Source: CAD feature listing. Evaluate the final solid. Frame: model axes, mm. Face numbers are marked on the shaded views. A direction names the side the tool comes from. Round coordinates to 2 decimals unless told otherwise and drop trailing zeros. Write each loop counter-clockwise with the first axis right and the second up, starting at its lowest first coordinate (ties: lowest second). Pieces come first, ordered by that corner, then holes.
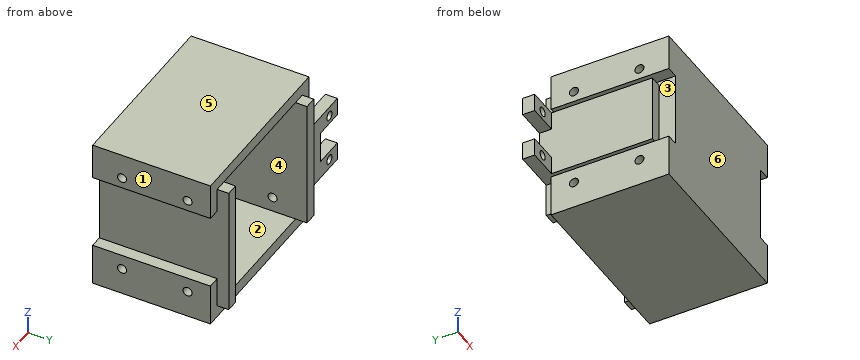
```python
from build123d import *

# Parameters (mm, degrees)
BOSS_EXTRUDE1_DEPTH      = 43
SKETCH4_W                = 50.5
SKETCH4_H                = 39.147537046
BOSS_EXTRUDE2_DEPTH      = 4
SKETCH5_W                = 50.5
SKETCH5_H                = 39.147537046
BOSS_EXTRUDE3_DEPTH      = 4
BOSS_EXTRUDE4_DEPTH      = 17.5
BOSS_EXTRUDE4_DEPTH_BACK = 16
BOSS_EXTRUDE5_START      = 17.5
SKETCH3_3_W              = 10
SKETCH3_3_H              = 6
SKETCH3_3_R              = 1.5
BOSS_EXTRUDE5_DEPTH      = 4
BOSS_EXTRUDE5_2_DEPTH    = 4
BOSS_EXTRUDE6_START      = 17.5
BOSS_EXTRUDE6_DEPTH      = 4
BOSS_EXTRUDE7_DEPTH      = 4
BOSS_EXTRUDE7_DEPTH_BACK = 10
SKETCH5_3_W              = 4
SKETCH5_3_H              = 39.147537046
BOSS_EXTRUDE8_DEPTH      = 4
BOSS_EXTRUDE8_DEPTH_BACK = 8
SKETCH8_R                = 1.5
CUT_EXTRUDE1_DEPTH       = 79.060873682
SKETCH11_R               = 1.5
CUT_EXTRUDE2_DEPTH       = 79.060873682


with BuildPart() as part:
    # Sketch1 → Boss-Extrude1 (new body)
    with BuildSketch(Plane.XY):
        Polygon((-21.25, -17.493697991), (-21.25, 21.493697991), (-25.25, 21.493697991), (-25.25, -21.493697991), (25.25, -21.493697991), (25.25, 21.493697991), (21.25, 21.493697991), (21.25, -17.493697991), align=None)
    extrude(amount=BOSS_EXTRUDE1_DEPTH)

    # Sketch4 → Boss-Extrude2 (add)
    with BuildSketch(Plane.XY.offset(43)):
        with Locations((0, -1.919929468)):
            Rectangle(SKETCH4_W, SKETCH4_H)
    extrude(amount=BOSS_EXTRUDE2_DEPTH)

    # Sketch5 → Boss-Extrude3 (add)
    with BuildSketch(Plane(origin=(0, 0, 0), x_dir=(-1, 0, 0), z_dir=(0, 0, -1))):
        with Locations((0, -1.919929468)):
            Rectangle(SKETCH5_W, SKETCH5_H)
    extrude(amount=BOSS_EXTRUDE3_DEPTH)


with BuildPart() as boss_extrude4_tool:
    # Sketch3 → Boss-Extrude4 (new, two sides: drawn at the far end of the back side and taken through both)
    with BuildSketch(Plane(origin=(0, 0, 0), x_dir=(1, 0, 0), z_dir=(0, 1, 0)).offset(-BOSS_EXTRUDE4_DEPTH_BACK)):
        Polygon((-29.250003781, -33.625807881), (-25.250003781, -33.625807881), (-25.250003781, -11.171909281), (-29.250003781, -11.171909281), (-29.250003781, -17.171909281), (-29.250003781, -27.625807881), align=None)
    extrude(amount=BOSS_EXTRUDE4_DEPTH + BOSS_EXTRUDE4_DEPTH_BACK)


with BuildPart() as part_1:
    add(part.part)


with BuildPart() as part_2:
    # Boss-Extrude4: joined with boss_extrude4_tool
    add(part_1.part.fuse(boss_extrude4_tool.part, tol=0.00001))


with BuildPart() as body_2:
    # Sketch3<3> → Boss-Extrude5 (new body)
    with BuildSketch(Plane(origin=(0, 0, 0), x_dir=(1, 0, 0), z_dir=(0, 1, 0)).offset(BOSS_EXTRUDE5_START)):
        with Locations((-34.250003781, -30.625807881)):
            Rectangle(SKETCH3_3_W, SKETCH3_3_H)
        with Locations(Location((-34.536906803, -30.406566851, 0), (0, 0, 270))):
            Circle(SKETCH3_3_R, mode=Mode.SUBTRACT)
    extrude(amount=BOSS_EXTRUDE5_DEPTH)


with BuildPart() as body_3:
    # Sketch3<3> → Boss-Extrude5 2 (new body)
    with BuildSketch(Plane(origin=(0, 0, 0), x_dir=(1, 0, 0), z_dir=(0, 1, 0)).offset(BOSS_EXTRUDE5_START)):
        with Locations((-34.250003781, -14.171909281)):
            Rectangle(SKETCH3_3_W, SKETCH3_3_H)
        with Locations(Location((-34.536906803, -14.310361699, 0), (0, 0, 270))):
            Circle(SKETCH3_3_R, mode=Mode.SUBTRACT)
    extrude(amount=BOSS_EXTRUDE5_2_DEPTH)


with BuildPart() as boss_extrude6_tool:
    # Sketch3<4> → Boss-Extrude6 (new body)
    with BuildSketch(Plane(origin=(0, 0, 0), x_dir=(1, 0, 0), z_dir=(0, 1, 0)).offset(BOSS_EXTRUDE6_START)):
        Polygon((-29.250003781, -33.625807881), (-25.250003781, -33.625807881), (-25.250003781, -11.171909281), (-29.250003781, -11.171909281), (-29.250003781, -17.171909281), (-29.250003781, -27.625807881), align=None)
    extrude(amount=BOSS_EXTRUDE6_DEPTH)


with BuildPart() as part_3:
    add(part_2.part)


with BuildPart() as part_4:
    # Boss-Extrude6: joined with boss_extrude6_tool
    add(part_3.part.fuse(boss_extrude6_tool.part, body_2.part, body_3.part, tol=0.00001))

    # Sketch5<3> → Boss-Extrude7 (add, two sides: drawn at the far end of the back side and taken through both)
    with BuildSketch(Plane(origin=(0, 0, 0), x_dir=(-1, 0, 0), z_dir=(0, 0, -1)).offset(-BOSS_EXTRUDE7_DEPTH_BACK)):
        with Locations((-27.25, -1.919929468)):
            Rectangle(SKETCH5_3_W, SKETCH5_3_H)
        with Locations((27.25, -1.919929468)):
            Rectangle(SKETCH5_3_W, SKETCH5_3_H)
    extrude(amount=BOSS_EXTRUDE7_DEPTH + BOSS_EXTRUDE7_DEPTH_BACK)

    # Sketch4<3> → Boss-Extrude8 (add, two sides: drawn at the far end of the back side and taken through both)
    with BuildSketch(Plane.XY.offset(43).offset(-BOSS_EXTRUDE8_DEPTH_BACK)):
        Polygon((29.25, 17.653839055), (25.25, 17.653839055), (25.25, -21.493697991), (29.25, -21.493697991), (29.25, -17.493697991), (29.25, 13.653839055), align=None)
        Polygon((-25.25, -21.493697991), (-25.25, 17.653839055), (-29.25, 17.653839055), (-29.25, 13.653839055), (-29.25, -17.493697991), (-29.25, -21.493697991), align=None)
    extrude(amount=BOSS_EXTRUDE8_DEPTH + BOSS_EXTRUDE8_DEPTH_BACK)

    # Sketch8 → Cut-Extrude1 (cut, through all)
    with BuildSketch(Plane.ZY.offset(29.25)):
        with Locations((5.005736184, 10.04444872)):
            Circle(SKETCH8_R)
        with Locations((5.005736184, -11.726773354)):
            Circle(SKETCH8_R)
    extrude(amount=-CUT_EXTRUDE1_DEPTH, mode=Mode.SUBTRACT)

    # Sketch11 → Cut-Extrude2 (cut, through all)
    with BuildSketch(Plane.ZY.offset(29.25)):
        with Locations((38.59734476, -11.726773354)):
            Circle(SKETCH11_R)
        with Locations((38.59734476, 10.04444872)):
            Circle(SKETCH11_R)
    extrude(amount=-CUT_EXTRUDE2_DEPTH, mode=Mode.SUBTRACT)


solid = part_4.part
```
Q1. Section query B-B, the plane y = 3. Output: boundary loops of the cut face in (x, z), and give its area (3 significant figures).
Q2. Set-up query: the marked faces 1 and 2. Return all of +Z, -Z, +X, -X, +Y, -Y with unobstructed straight access to the full face (end or side cutting, diameter ignored); none if empty.
Q3. Mould query, pull axis Z, two halves, no side actions, for the marked faces 3, 4, 5 and 6. Classes: pulls with the +Z half, pulls with the -Z half, needs draft (parallel to the pull), parting line crosses it, or undercut.
Q4. Pin query (flat end, axial travel): P1, Ø10, axis at x = -18.5, z = 36, coming from the +Y side; P2, Ø7, axis at x = -6, z = 5.5, coming from the +Y side; P3, Ø10, axis at y = 3, z = 22, coming from the -X side. Return the tip coordinate at first contact, or that it passes through.
Q5. Section query D-D, the plane x = 16. Output: boundary loops of the cut face in (y, z).
Q6. Section query C-C, the plane z = 41.5. Output: boundary loops of the cut face in (x, y), and give its area (3 significant figures).
Q7. Line query: line 1 (Z direction, x = 18, y = 0); line 2 (X direction, y = 16.5, z = 19); line 3 (Z direction, x = -27.5, y = 12). Output: solid intervals per line, ascending.
Q8. Section query A-A, the plane x = -32. Output: boundary loops of the cut face in (y, z), and give its area (3 significant figures).
Filled in:
1. outline: (-29.25, -4) - (29.25, -4) - (29.25, 10) - (25.25, 10) - (25.25, 35) - (29.25, 35) - (29.25, 47) - (-29.25, 47) - (-29.25, 35) - (-25.25, 35) - (-25.25, 33.63) - (-29.25, 33.63) - (-29.25, 11.17) - (-25.25, 11.17) - (-25.25, 10) - (-29.25, 10) - close; hole (-21.25, 0) - (21.25, 0) - (21.25, 43) - (-21.25, 43) - close
1. area: 1,050 mm2
2. face 1: +Z, -Z, +X, +Y, -Y
2. face 2: +Y
3. face 3: undercut
3. face 4: undercut
3. face 5: pulls with the +Z half
3. face 6: needs draft
4. P1: stops at y = 21.49
4. P2: stops at y = -17.49
4. P3: stops at x = -29.25
5. outline: (-21.49, -4) - (17.65, -4) - (17.65, 0) - (-17.49, 0) - (-17.49, 43) - (17.65, 43) - (17.65, 47) - (-21.49, 47) - close
6. outline: (-29.25, -21.49) - (29.25, -21.49) - (29.25, 17.65) - (25.25, 17.65) - (25.25, 21.49) - (21.25, 21.49) - (21.25, -17.49) - (-21.25, -17.49) - (-21.25, 21.49) - (-25.25, 21.49) - (-25.25, 17.65) - (-29.25, 17.65) - close
6. area: 827 mm2
7. line 1: z = -4 to 0, 43 to 47
7. line 2: x = -29.25 to -21.25, 21.25 to 25.25
7. line 3: z = -4 to 10, 11.17 to 33.63, 35 to 47
8. outline: (17.5, 11.17) - (21.5, 11.17) - (21.5, 17.17) - (17.5, 17.17) - close; (17.5, 27.63) - (21.5, 27.63) - (21.5, 33.63) - (17.5, 33.63) - close
8. area: 48.0 mm2
